```python
from build123d import *

# Parameters (mm, degrees)
BOSS_EXTRUDE1_DEPTH      = 30
BOSS_EXTRUDE1_DEPTH_BACK = 30
SKETCH2_R                = 3.25
SKETCH2_R_2              = 1.25
SKETCH2_R_3              = 5
SKETCH3_W                = 58
SKETCH3_H                = 55
CUT_EXTRUDE1_DEPTH       = 60.373815778
SKETCH4_W                = 10
SKETCH4_H                = 8
BOSS_EXTRUDE2_DEPTH      = 10
FILLET1_R                = 4
SKETCH5_R                = 1.75
CUT_EXTRUDE2_DEPTH       = 76.599272483
FILLET1_OF_MIRROR1_R     = 4
FILLET2_R                = 4
SKETCH6_R                = 1.25
SKETCH6_R_2              = 5
BOSS_EXTRUDE3_DEPTH      = 3
SKETCH7_R                = 2.5
CUT_EXTRUDE3_DEPTH       = 2
SKETCH8_R                = 2
CUT_EXTRUDE4_DEPTH       = 62.36774397


with BuildPart() as part:
    # Sketch2 → Boss-Extrude1 (new, two sides: drawn at the far end of the back side and taken through both)
    with BuildSketch(Plane.XY.offset(-BOSS_EXTRUDE1_DEPTH_BACK)):
        with BuildLine():
            Line((-7.5, 5), (-7.5, 30))
            Line((-7.5, 30), (5.086494468, 45))
            Line((5.086494468, 45), (24.5, 45))
            Line((24.5, 45), (24.5, 20))
            Line((24.5, 20), (7.5, 20))
            Line((7.5, 20), (7.5, 5))
            ThreePointArc((7.5, 5), (6.035533906, 1.464466094), (2.5, 0))
            Line((2.5, 0), (-2.5, 0))
            ThreePointArc((-2.5, 0), (-6.035533906, 1.464466094), (-7.5, 5))
        make_face()
        with Locations((0, 5)):
            Circle(SKETCH2_R, mode=Mode.SUBTRACT)
        with Locations((18.004770913, 32.569673822)):
            Circle(SKETCH2_R_2, mode=Mode.SUBTRACT)
        with Locations((-0.995229087, 32.569673822)):
            Circle(SKETCH2_R_2, mode=Mode.SUBTRACT)
        with Locations((8.504770913, 29.569673822)):
            Circle(SKETCH2_R_3, mode=Mode.SUBTRACT)
    extrude(amount=BOSS_EXTRUDE1_DEPTH + BOSS_EXTRUDE1_DEPTH_BACK)

    # Sketch3 → Cut-Extrude1 (cut, through all)
    with BuildSketch(Plane(origin=(0, 45, 0), x_dir=(1, 0, 0), z_dir=(0, 1, 0))):
        with Locations((-7.5, 0)):
            Rectangle(SKETCH3_W, SKETCH3_H)
    extrude(amount=-CUT_EXTRUDE1_DEPTH, mode=Mode.SUBTRACT)

    # Sketch4 → Boss-Extrude2 (add)
    with BuildSketch(Plane(origin=(24.5, 0, 0), x_dir=(0, 0, -1), z_dir=(1, 0, 0))):
        with Locations((-25, 41)):
            Rectangle(SKETCH4_W, SKETCH4_H)
    boss_extrude2 = extrude(amount=BOSS_EXTRUDE2_DEPTH)

    # Fillet1
    fillet1_edges = [part.edges().sort_by_distance(p)[0] for p in [
        (34.5, 37, 25),
        (34.5, 45, 25),
    ]]
    fillet(fillet1_edges, radius=FILLET1_R - 0.0001)  # a hair under: the kernel refuses the full size

    # Sketch5 → Cut-Extrude2 (cut, through all)
    with BuildSketch(Plane(origin=(0, 0, 20), x_dir=(-1, 0, 0), z_dir=(0, 0, -1))):
        with Locations((-30.5, 41)):
            Circle(SKETCH5_R)
    cut_extrude2 = extrude(amount=-CUT_EXTRUDE2_DEPTH, mode=Mode.SUBTRACT)

    # Mirror1: Boss-Extrude2, Cut-Extrude2 across plane
    add(boss_extrude2.mirror(Plane.XY))
    add(cut_extrude2.mirror(Plane.XY), mode=Mode.SUBTRACT)

    # Fillet1 of Mirror1
    fillet1_of_mirror1_edges = [part.edges().sort_by_distance(p)[0] for p in [
        (34.5, 37, -25),
        (34.5, 45, -25),
    ]]
    fillet(fillet1_of_mirror1_edges, radius=FILLET1_OF_MIRROR1_R - 0.0001)  # a hair under: the kernel refuses the full size

    # Fillet2
    fillet2_edges = [part.edges().sort_by_distance(p)[0] for p in [
        (24.5, 37, 25),
        (24.5, 41, 20),
        (24.5, 37, -25),
        (24.5, 41, -20),
        (5.086494468, 45, -28.75),
        (7.5, 20, -28.75),
        (-7.5, 30, -28.75),
        (-7.5, 30, 28.75),
        (7.5, 20, 28.75),
        (5.086494468, 45, 28.75),
    ]]
    fillet(fillet2_edges, radius=FILLET2_R)

    # Sketch6 → Boss-Extrude3 (add)
    with BuildSketch(Plane.XY.offset(-27.5)):
        with BuildLine():
            Line((21.5, 45), (6.9517251, 45))
            ThreePointArc((6.9517251, 45), (5.261252053, 44.625231148), (3.887547328, 43.571150439))
            Line((3.887547328, 43.571150439), (-6.564177772, 31.115269502))
            ThreePointArc((-6.564177772, 31.115269502), (-7.258770483, 29.912199636), (-7.5, 28.544119063))
            ThreePointArc((-7.5, 28.544119063), (0.776489044, 21.551274863), (11.5, 20))
            Line((11.5, 20), (21.5, 20))
            Line((21.5, 20), (21.5, 45))
        make_face()
        with Locations((18.004770913, 32.569673822)):
            Circle(SKETCH6_R, mode=Mode.SUBTRACT)
        with Locations((8.504770913, 29.569673822)):
            Circle(SKETCH6_R_2, mode=Mode.SUBTRACT)
        with Locations((-0.995229087, 32.569673822)):
            Circle(SKETCH6_R, mode=Mode.SUBTRACT)
    boss_extrude3 = extrude(amount=BOSS_EXTRUDE3_DEPTH)

    # Sketch7 → Cut-Extrude3 (cut)
    with BuildSketch(Plane(origin=(0, 0, -30), x_dir=(-1, 0, 0), z_dir=(0, 0, -1))):
        with Locations((-18.004770913, 32.569673822)):
            Circle(SKETCH7_R)
        with Locations((0.995229087, 32.569673822)):
            Circle(SKETCH7_R)
    cut_extrude3 = extrude(amount=-CUT_EXTRUDE3_DEPTH, mode=Mode.SUBTRACT)

    # Mirror2: Boss-Extrude3, Cut-Extrude3 across plane
    add(boss_extrude3.mirror(Plane.XY))
    add(cut_extrude3.mirror(Plane.XY), mode=Mode.SUBTRACT)

    # Sketch8 → Cut-Extrude4 (cut, through all)
    with BuildSketch(Plane.ZY.offset(-21.5)):
        with Locations((0, 26)):
            Circle(SKETCH8_R)
    extrude(amount=-CUT_EXTRUDE4_DEPTH, mode=Mode.SUBTRACT)


solid = part.part
```
Source: CAD feature listing. Evaluate the final solid. Frame: model axes, mm. A direction names the side the tool comes from. Round coordinates to 2 decimals unless told otherwise and drop trailing zeros. Loops run counter-clockwise (first coordinate to the right, second up) from the corner with the lowest first, then second, coordinate; pieces in that order, holes last. Notation, with made-up numbers: M 70.5,-36 L 110.5,-36 A11 cw 110.5,-21 Z; hole C 5.5,-22 d7. An arc over 180 degrees is marked long. Put each result on its own line as item: value.
(1) Ray query, line 1 (Z direction, x = 1.5, y = 25.5); line 2 (Y direction, x = 0, z = 28.8); line 3 (Y direction, x = 30.5, z = -25.75). Return the intervals inside material, ascending. Write a range as [from, to].
Solutions:
line 1: [-30, -24.5], [24.5, 30]
line 2: [0, 1.75], [8.25, 30.28], [34.86, 38.94]
line 3: [37, 39.25], [42.75, 45]
(2) Section C-C, the plane y = 26. Return loops of the section in (x, z), and give its area (3 significant figures).
Solutions:
outline: M -7.5,-30 L 5,-30 L 5,-24.5 L -5.47,-24.5 L -5.47,-27.5 L -7.5,-27.5 Z; M -7.5,27.5 L -5.47,27.5 L -5.47,24.5 L 5,24.5 L 5,30 L -7.5,30 Z; M 12.01,-30 L 24.5,-30 L 24.5,-2 L 21.5,-2 L 21.5,-24.5 L 12.01,-24.5 Z; M 12.01,24.5 L 21.5,24.5 L 21.5,2 L 24.5,2 L 24.5,30 L 12.01,30 Z
area: 398 mm²
(3) Access query for faces 1 (the face through (16.851, 30.352, -29.014)), 2 (the face through (7.5, 11, -29)), 3 (the face through (-1, 11, -27.5)), 4 (the face through (17.73, 31.35, -26.27)). Directions: +Z, -Z, +X, -X, +Y, -Y. A direction counts if a zero-diameter tool reaches every point of the face in a straight line with its end or side. Return the directions, or none.
Solutions:
face 1: -Z
face 2: +Z, -Z, +X, -Y
face 3: -X, -Y
face 4: +Z, -Z
(4) Section D-D, the plane y = 36. Return loops of the section in (x, z).
Solutions:
outline: M -2.47,-30 L 25.85,-30 L 25.85,-19 A4 cw 24.5,-16 L 24.5,16 A4 cw 25.85,19 L 25.85,30 L -2.47,30 L -2.47,24.5 L 21.5,24.5 L 21.5,-24.5 L -2.47,-24.5 Z
(5) Section A-A, the plane y = 11. Return loops of the section in (x, z).
Solutions:
outline: M -7.5,-30 L 7.5,-30 L 7.5,-27.5 L -7.5,-27.5 Z; M -7.5,27.5 L 7.5,27.5 L 7.5,30 L -7.5,30 Z
(6) Pull-direction query (X, two-part tool) for faces 5 (the face through (13, 27, -30)), 6 (the face through (25.641, 35.797, 24.458)), 7 (the face through (-2, 34, 28)); classes: released by +X, released by -X, zero draft, split by the parting line, or undercut.
Solutions:
face 5: zero draft
face 6: released by +X
face 7: undercut
(7) Section B-B, the plane z = 0. Return loops of the section in (x, y), and give its area (3 significant figures).
Solutions:
outline: M 21.5,20 L 24.5,20 L 24.5,24 L 21.5,24 Z; M 21.5,28 L 24.5,28 L 24.5,45 L 21.5,45 Z
area: 63.0 mm²
(8) First-contact query: pin 1 (6 mm diameter, centred on y = 39.5, z = -7.5, fed in from -X); pin 2 (3 mm diameter, centred on x = 20.5, z = -17, fed in from -Y); pin 3 (1.6 mm diameter, centred on x = 29, z = -23, fed in from -Y). Flat tips, straight axial feed; report the tip coordinate or a pass-through.
Solutions:
pin 1: x = 21.5
pin 2: y = 20
pin 3: y = 36.99
